from build123d import *

# Parameters (mm, degrees)
SKETCH2_R                 = 24.13
SKETCH2_R_2               = 6.35
BOSS_EXTRUDE1_DEPTH       = 5.7658
SKETCH10_W                = 12.7
SKETCH10_H                = 3.175
CUT_EXTRUDE2_DEPTH        = 5.7658
F_4_CLEARANCE_HOLE2_D     = 2.9464
F_4_CLEARANCE_HOLE2_DEPTH = 5.7668
CIRPATTERN2_COUNT         = 4
BOSS_EXTRUDE2_DEPTH       = 5.7658
BOSS_EXTRUDE4_DEPTH       = 5.7658
F_4_CLEARANCE_HOLE3_D     = 2.9464
F_4_CLEARANCE_HOLE3_DEPTH = 5.7658
BOSS_EXTRUDE3_DEPTH       = 5.7658
CUT_EXTRUDE4_REACH        = 7.766
SKETCH30_W                = 10.8839
SKETCH30_H                = 33.094
FILLET2_R                 = 1.524


with BuildPart() as part:
    # Sketch2 → Boss-Extrude1 (new body)
    with BuildSketch(Plane(origin=(0, 0, 0), x_dir=(1, 0, 0), z_dir=(0, 1, 0))):
        Circle(SKETCH2_R)
        Circle(SKETCH2_R_2, mode=Mode.SUBTRACT)
    extrude(amount=BOSS_EXTRUDE1_DEPTH)

    # Sketch10 → Cut-Extrude2 (cut)
    with BuildSketch(Plane(origin=(0, 5.7658, 0), x_dir=(1, 0, 0), z_dir=(0, 1, 0))):
        with Locations((0, 14.2875)):
            Rectangle(SKETCH10_W, SKETCH10_H)
    cut_extrude2 = extrude(amount=-CUT_EXTRUDE2_DEPTH, mode=Mode.SUBTRACT)

    # #4 Clearance Hole2
    with Locations(Plane(origin=(0, 5.7658, 0), x_dir=(1, 0, 0), z_dir=(0, 1, 0))):
        with Locations((0, 9.525)):
            f_4_clearance_hole2 = Hole(F_4_CLEARANCE_HOLE2_D / 2, depth=F_4_CLEARANCE_HOLE2_DEPTH)

    # CirPattern2: Cut-Extrude2, #4 Clearance Hole2 ×4 about axis
    cirpattern2_axis = Axis((0, 0, 0), (0, 1, 0))
    for i in range(1, CIRPATTERN2_COUNT):
        add(cut_extrude2.rotate(cirpattern2_axis, i * 360 / CIRPATTERN2_COUNT), mode=Mode.SUBTRACT)
        add(f_4_clearance_hole2.rotate(cirpattern2_axis, i * 360 / CIRPATTERN2_COUNT), mode=Mode.SUBTRACT)

    # Sketch16 → Boss-Extrude2 (add)
    with BuildSketch(Plane(origin=(0, 5.7658, 0), x_dir=(1, 0, 0), z_dir=(0, 1, 0))):
        with BuildLine():
            Line((-24.13, 0), (-24.13, -27.721453785))
            Line((-24.13, -27.721453785), (-32.893, -37.084))
            Line((-32.893, -37.084), (-32.893, -91.174))
            Line((-32.893, -91.174), (32.893, -91.174))
            Line((32.893, -91.174), (32.893, -37.084))
            Line((32.893, -37.084), (24.13, -27.721453785))
            Line((24.13, -27.721453785), (24.13, 0))
            ThreePointArc((24.13, 0), (21.910168678, -10.109471228), (15.6591, -18.358907571))
            Line((15.6591, -18.358907571), (15.6591, -37.084))
            Line((15.6591, -37.084), (20.193, -37.084))
            Line((20.193, -37.084), (20.193, -58.674))
            Line((20.193, -58.674), (20.193, -78.474))
            Line((20.193, -78.474), (-20.193, -78.474))
            Line((-20.193, -78.474), (-20.193, -58.674))
            Line((-20.193, -58.674), (-20.193, -37.084))
            Line((-20.193, -37.084), (-15.6591, -37.084))
            Line((-15.6591, -37.084), (-15.6591, -18.358907571))
            ThreePointArc((-15.6591, -18.358907571), (-21.910168678, -10.109471228), (-24.13, 0))
        make_face()
    extrude(amount=-BOSS_EXTRUDE2_DEPTH)

    # Sketch32 → Boss-Extrude4 (add)
    with BuildSketch(Plane(origin=(0, 5.7658, 0), x_dir=(1, 0, 0), z_dir=(0, 1, 0))):
        with BuildLine():
            ThreePointArc((15.6591, -18.358907571), (8.344353159, -22.64130452), (-6.7e-08, -24.13))
            Line((-6.7e-08, -24.13), (15.6591, -24.13))
            Line((15.6591, -24.13), (15.6591, -18.358907571))
        make_face()
        with BuildLine():
            Line((-15.6591, -18.358907571), (-15.6591, -24.13))
            Line((-15.6591, -24.13), (-6.7e-08, -24.13))
            ThreePointArc((-6.7e-08, -24.13), (-8.344353221, -22.641304497), (-15.6591, -18.358907571))
        make_face()
    extrude(amount=-BOSS_EXTRUDE4_DEPTH)

    # #4 Clearance Hole3
    with Locations(Plane(origin=(0, 5.7658, 0), x_dir=(1, 0, 0), z_dir=(0, 1, 0))):
        with Locations((-24.2, -63.574), (-24.2, -73.574), (24.2, -63.574), (24.2, -73.574)):
            Hole(F_4_CLEARANCE_HOLE3_D / 2, depth=F_4_CLEARANCE_HOLE3_DEPTH)

    # Sketch31 → Boss-Extrude3 (add)
    with BuildSketch(Plane(origin=(0, 5.7658, 0), x_dir=(1, 0, 0), z_dir=(0, 1, 0))):
        Polygon((-32.893, -37.084), (-32.893, -24.384), (-24.13, -15.021453785), (-24.13, -27.721453785), align=None)
    extrude(amount=-BOSS_EXTRUDE3_DEPTH)

    # Sketch30 → Cut-Extrude4 (cut, up to next)
    with BuildSketch(Plane(origin=(0, 5.7658, 0), x_dir=(1, 0, 0), z_dir=(0, 1, 0)), mode=Mode.PRIVATE) as cut_extrude4_sk1:
        with Locations((-21.10105, -40.677)):
            Rectangle(SKETCH30_W, SKETCH30_H)
    cut_extrude4_tool1 = extrude(cut_extrude4_sk1.sketch, amount=-CUT_EXTRUDE4_REACH, mode=Mode.PRIVATE) & part.part
    add(cut_extrude4_tool1.solids().sort_by_distance((-21.10105, 5.7658, 40.677))[0], mode=Mode.SUBTRACT)

    # Fillet2
    fillet2_edges = [part.edges().sort_by_distance(p)[0] for p in [
        (15.6591, 2.8829, 24.13),
        (-26.543, 2.8829, 57.224),
        (-26.543, 2.8829, 24.13),
        (-20.193, 2.8829, 57.224),
        (-20.193, 2.8829, 78.474),
        (20.193, 2.8829, 78.474),
        (20.193, 2.8829, 37.084),
        (15.6591, 2.8829, 37.084),
    ]]
    fillet(fillet2_edges, radius=FILLET2_R)


solid = part.part
Here's how the part is built. I have some questions about the finished solid (model axes, mm). Round coordinates to 2 decimals unless told otherwise and drop trailing zeros. Loops run counter-clockwise (first coordinate to the right, second up) from the corner with the lowest first, then second, coordinate; pieces in that order, holes last. Notation, with made-up numbers: (-6, -6) - (45, -6) arc R8 cw to (45, 9) - close; hole circle Ø6 at (46, 57). An arc over 180 degrees is marked (long way). One line per question, with ' | ' between items. Start each with the question number.
Q1. Please list where these lines run through material, in increasing order: line 1 (Z direction, x = -4.5, y = 2.65) (3 decimals); line 2 (Z direction, x = -14, y = 1.65); line 3 (X direction, y = 3.75, z = 45). Write a range as [from, to].
Q2. I want a section at D-D (y = 4.9). State how many separate pieces and enclosed holes the cut face has, then the cut area to 3 significant figures.
Q3. I want a section at B-B (z = 52). Write out the boundary of the cut face in (x, y).
Q4. I want a section at C-C (x = -14.5). Write out the boundary of the cut face in (y, z), then the cut area to 3 significant figures.
Q5. Will these pins go through, and if not, where does the flat tip stop? pin 1 (2.5 mm diameter, centred on y = 1.5, z = 14, fed in from -X); pin 2 (1.5 mm diameter, centred on y = 4.5, z = 3.5, fed in from +X); pin 3 (2.5 mm diameter, centred on x = -14, y = 1.5, fed in from -Z).
Q6. We'd pull the mould along X, two halves only. Please class faces 1 (the flat face through (15.659, 3, 31)), 2 (the flat face through (24.13, 3, 14)): +X half, -X half, draft (parallel to the pull), parting line (faces both ways), or undercut.
Q7. I want a section at A-A (x = 0). Write out the boundary of the cut face in (y, z) (3 decimals).
Response values:
1) line 1: z = [-23.707, -15.875], [-12.7, -4.48], [4.48, 12.7], [15.875, 24.13], [78.474, 91.174] | line 2: z = [-19.65, -6.35], [6.35, 24.13], [78.47, 91.17] | line 3: x = [-32.89, -26.54], [20.19, 32.89]
2) separate pieces: 1 | enclosed holes: 14 | area: 3,770 mm²
3) outline: (-32.89, 0) - (-26.54, 0) - (-26.54, 5.77) - (-32.89, 5.77) - close; (20.19, 0) - (32.89, 0) - (32.89, 5.77) - (20.19, 5.77) - close
4) outline: (0, -19.29) - (5.77, -19.29) - (5.77, -6.35) - (0, -6.35) - close; (0, 6.35) - (5.77, 6.35) - (5.77, 24.13) - (0, 24.13) - close; (0, 78.47) - (5.77, 78.47) - (5.77, 91.17) - (0, 91.17) - close | area: 250 mm²
5) pin 1: stops at x = -24.34 | pin 2: stops at x = 24.13 | pin 3: stops at z = -20.49
6) face 1: undercut | face 2: +X half
7) outline: (0, -24.13) - (5.766, -24.13) - (5.766, -15.875) - (0, -15.875) - close; (0, -12.7) - (5.766, -12.7) - (5.766, -10.998) - (0, -10.998) - close; (0, -8.052) - (5.766, -8.052) - (5.766, -6.35) - (0, -6.35) - close; (0, 6.35) - (5.766, 6.35) - (5.766, 8.052) - (0, 8.052) - close; (0, 10.998) - (5.766, 10.998) - (5.766, 12.7) - (0, 12.7) - close; (0, 15.875) - (5.766, 15.875) - (5.766, 24.13) - (0, 24.13) - close; (0, 78.474) - (5.766, 78.474) - (5.766, 91.174) - (0, 91.174) - close
